Work out the finished part from the listing and answer in its coordinate system (mm). Face numbers are marked on the shaded views. Give positions to 0.01 mm unless a question says otherwise; leave off trailing zeros. Order: outer loops, then holes, each group sorted by start corner. A loop starts at its lowest first (then second) coordinate and runs counter-clockwise, first axis right, second up.
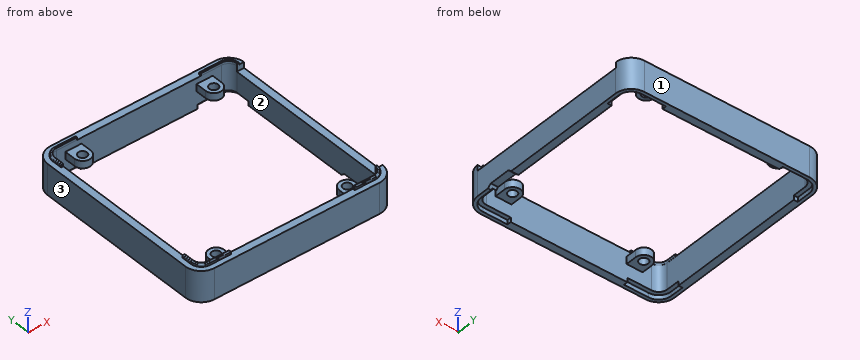
```python
from build123d import *

# Parameters (mm, degrees)
EXTRUDE006_DEPTH                     = 2
EXTRUDE006_ONTO_SKETCH006_ROLL_ANGLE = 90
EXTRUDE006_PLACEMENT_ANGLE           = 90
SKETCH_W                             = 14.047477
SKETCH_H                             = 45.6
EXTRUDE004_DEPTH                     = 10
SKETCH002_R                          = 1.2
EXTRUDE001_DEPTH                     = 2
EXTRUDE005_DEPTH                     = 10
EXTRUDE003_DEPTH                     = 0.7
EXTRUDE003_DEPTH_BACK                = 0.2
FILLET_R                             = 0.2
CHAMFER_SIZE                         = 0.2
EXTRUDE002_DEPTH                     = 2
EXTRUDE_DEPTH                        = 1.6
EXTRUDE_DEPTH_BACK                   = 6.8


with BuildPart() as extrude006:
    # Sketch006 as drawn → Extrude006 (new, symmetric)
    with BuildSketch(Plane.XY):
        Polygon((-3.8, 0), (-2.9, 0.8), (2.9, 0.8), (3.8, 0), align=None)
    extrude(amount=EXTRUDE006_DEPTH, both=True)


with BuildPart() as extrude006_1:
    # Extrude006 onto Sketch006 roll: moved
    add(extrude006.part.rotate(Axis((0, 0, 0), (1, 0, 0)), EXTRUDE006_ONTO_SKETCH006_ROLL_ANGLE))


with BuildPart() as extrude006_2:
    # Extrude006 onto Sketch006 placement: moved
    add(extrude006_1.part)


with BuildPart() as extrude006_3:
    # Extrude006 placement: moved
    add(extrude006_2.part.moved(Location((50, 9.5, -6.8))).rotate(Axis((50, 9.5, -6.8), (0, 0, 1)), EXTRUDE006_PLACEMENT_ANGLE))


with BuildPart() as extrude004:
    # Sketch → Extrude004 (new body)
    with BuildSketch(Plane.XY):
        with Locations((51.252235, 25)):
            Rectangle(SKETCH_W, SKETCH_H)
    extrude(amount=EXTRUDE004_DEPTH)


with BuildPart() as extrude001:
    # Sketch002 → Extrude001 (new body)
    with BuildSketch(Plane.XY):
        with BuildLine():
            Line((4.8, 47), (4.8, 51))
            Line((4.8, 51), (9.2, 51))
            Line((9.2, 51), (9.2, 47.000001))
            ThreePointArc((4.8, 47), (7, 44.8), (9.2, 47.000001))
        make_face()
        with Locations((7, 47)):
            Circle(SKETCH002_R, mode=Mode.SUBTRACT)
        with BuildLine():
            ThreePointArc((9.2, 3), (7, 5.2), (4.8, 3))
            Line((4.8, 3), (4.8, -1))
            Line((4.8, -1), (9.2, -1))
            Line((9.2, -1), (9.2, 3))
        make_face()
        with Locations((7, 3)):
            Circle(SKETCH002_R, mode=Mode.SUBTRACT)
        with BuildLine():
            Line((40.8, 47), (40.8, 51))
            Line((40.8, 51), (45.2, 51))
            Line((45.2, 51), (45.2, 46.999987))
            ThreePointArc((40.8, 47), (42.999993, 44.8), (45.2, 46.999987))
        make_face()
        with Locations((43, 47)):
            Circle(SKETCH002_R, mode=Mode.SUBTRACT)
        with BuildLine():
            ThreePointArc((45.2, 3), (43, 5.2), (40.8, 3))
            Line((40.8, 3), (40.8, -1))
            Line((40.8, -1), (45.2, -1))
            Line((45.2, -1), (45.2, 3))
        make_face()
        with Locations((43, 3)):
            Circle(SKETCH002_R, mode=Mode.SUBTRACT)
    extrude(amount=-EXTRUDE001_DEPTH)


with BuildPart() as extrude005:
    # Sketch005 → Extrude005 (new body)
    with BuildSketch(Plane.XY):
        Polygon((8, 53), (8, 45), (-3, 45), (-3, 5), (8, 5), (8, -3), (42, -3), (42, 5), (53, 5), (53, 45), (42, 45), (42, 53), align=None)
    extrude(amount=EXTRUDE005_DEPTH)


with BuildPart() as cut003:
    # Sketch004 → Extrude003 (new body, two sides)
    with BuildSketch(Plane.XY) as extrude003_sk:
        with BuildLine():
            Line((2.3, 50.6), (47.7, 50.6))
            ThreePointArc((50.6, 47.7), (49.75061, 49.75061), (47.7, 50.6))
            Line((50.6, 47.7), (50.6, 2.3))
            ThreePointArc((47.7, -0.6), (49.75061, 0.24939), (50.6, 2.3))
            Line((47.7, -0.6), (2.3, -0.6))
            ThreePointArc((-0.6, 2.3), (0.24939, 0.24939), (2.3, -0.6))
            Line((-0.6, 2.3), (-0.6, 47.7))
            ThreePointArc((2.3, 50.6), (0.24939, 49.75061), (-0.6, 47.7))
        make_face()
        with BuildLine():
            Line((2.3, 50), (47.7, 50))
            ThreePointArc((50, 47.7), (49.326346, 49.326346), (47.7, 50))
            Line((50, 47.7), (50, 2.3))
            ThreePointArc((47.7, 0), (49.326346, 0.673654), (50, 2.3))
            Line((47.7, 0), (2.3, 0))
            ThreePointArc((0, 2.3), (0.673654, 0.673654), (2.3, 0))
            Line((0, 2.3), (0, 47.7))
            ThreePointArc((2.3, 50), (0.673654, 49.326346), (0, 47.7))
        make_face(mode=Mode.SUBTRACT)
    extrude(amount=EXTRUDE003_DEPTH)
    extrude(extrude003_sk.sketch, amount=-EXTRUDE003_DEPTH_BACK)


with BuildPart() as cut003_1:
    # Extrude003 placement: moved
    add(cut003.part.moved(Location((0, 0, 1.6))))

    # Fillet
    fillet_edges = [cut003_1.edges().sort_by_distance(p)[0] for p in [
        (-0.6, 25, 2.3),
        (0.24939, 49.75061, 2.3),
        (25, 50.6, 2.3),
        (49.75061, 49.75061, 2.3),
        (50.6, 25, 2.3),
        (49.75061, 0.24939, 2.3),
        (25, -0.6, 2.3),
        (0.24939, 0.24939, 2.3),
    ]]
    fillet(fillet_edges, radius=FILLET_R)

    # Chamfer
    chamfer_edges = [cut003_1.edges().sort_by_distance(p)[0] for p in [
        (0, 25, 1.4),
        (0.673654, 49.326346, 1.4),
        (25, 50, 1.4),
        (49.326346, 49.326346, 1.4),
        (50, 25, 1.4),
        (49.326346, 0.673654, 1.4),
        (25, 0, 1.4),
        (0.673654, 0.673654, 1.4),
    ]]
    chamfer(chamfer_edges, length=CHAMFER_SIZE)

    # Cut003: cut Extrude005
    add(extrude005.part, mode=Mode.SUBTRACT)


with BuildPart() as extrude002:
    # Sketch003 → Extrude002 (new body)
    with BuildSketch(Plane.XY):
        with BuildLine():
            Line((2.3, 51.1), (9, 51.1))
            Line((9, 44), (9, 51.1))
            Line((-1.1, 44), (9, 44))
            Line((-1.1, 44), (-1.1, 47.654452))
            ThreePointArc((2.3, 51.1), (-0.12032, 50.088024), (-1.1, 47.654452))
        make_face()
        with BuildLine():
            Line((51.1, 47.699699), (51.1, 44))
            Line((41, 44), (51.1, 44))
            Line((41, 51.1), (41, 44))
            Line((41, 51.1), (47.698586, 51.1))
            ThreePointArc((51.1, 47.699699), (50.103681, 50.104468), (47.698586, 51.1))
        make_face()
        with BuildLine():
            Line((47.6997, -1.1), (41, -1.1))
            Line((41, -1.1), (41, 6))
            Line((41, 6), (51.1, 6))
            Line((51.1, 6), (51.1, 2.297304))
            ThreePointArc((47.6997, -1.1), (50.103016, -0.105134), (51.1, 2.297304))
        make_face()
        with BuildLine():
            Line((-1.1, 2.300296), (-1.1, 6))
            Line((-1.1, 6), (9, 6))
            Line((9, 6), (9, -1.1))
            Line((9, -1.1), (2.294563, -1.1))
            ThreePointArc((-1.1, 2.300296), (-0.106103, -0.10205), (2.294563, -1.1))
        make_face()
    extrude(amount=-EXTRUDE002_DEPTH)


with BuildPart() as extrude002_1:
    # Extrude002 placement: moved
    add(extrude002.part.moved(Location((0, 0, -5.6))))


with BuildPart() as cut004:
    # Sketch001 → Extrude (new body, two sides)
    with BuildSketch(Plane.XY) as extrude_sk:
        with BuildLine():
            Line((2.3, 52), (47.7, 52))
            ThreePointArc((52, 47.7), (50.740559, 50.740559), (47.7, 52))
            Line((52, 47.7), (52, 2.3))
            ThreePointArc((47.7, -2), (50.740559, -0.740559), (52, 2.3))
            Line((47.7, -2), (2.3, -2))
            ThreePointArc((-2, 2.3), (-0.740559, -0.740559), (2.3, -2))
            Line((-2, 2.3), (-2, 47.7))
            ThreePointArc((2.3, 52), (-0.740559, 50.740559), (-2, 47.7))
        make_face()
        with BuildLine():
            Line((2.3, 50.01), (47.7, 50.01))
            ThreePointArc((50.01, 47.7), (49.333417, 49.333417), (47.7, 50.01))
            Line((50.01, 47.7), (50.01, 2.3))
            ThreePointArc((47.7, -0.01), (49.333417, 0.666583), (50.01, 2.3))
            Line((47.7, -0.01), (2.3, -0.01))
            ThreePointArc((-0.01, 2.3), (0.666583, 0.666583), (2.3, -0.01))
            Line((-0.01, 2.3), (-0.01, 47.7))
            ThreePointArc((2.3, 50.01), (0.666583, 49.333417), (-0.01, 47.7))
        make_face(mode=Mode.SUBTRACT)
    extrude(amount=EXTRUDE_DEPTH)
    extrude(extrude_sk.sketch, amount=-EXTRUDE_DEPTH_BACK)

    # Cut002: cut Extrude002
    add(extrude002_1.part, mode=Mode.SUBTRACT)

    # Fusion001: union Cut003
    add(cut003_1.part)

    # Fusion002: union Extrude001
    add(extrude001.part)

    # Cut: cut Extrude004
    add(extrude004.part, mode=Mode.SUBTRACT)

    # Cut004: cut Extrude006
    add(extrude006_3.part, mode=Mode.SUBTRACT)


solid = cut004.part
```
1. The part is cut by section A-A (x = 39.5). Write down the section's boundary in (y, z).
Findings below:
outline: (-2, -6.8) - (-0.01, -6.8) - (-0.01, 1.6) - (-2, 1.6) - close; (50.01, -6.8) - (52, -6.8) - (52, 1.6) - (50.01, 1.6) - close
2. The part is cut by section D-D (x = 7). State how many separate pieces and enclosed holes the cut face has, then the cut area to 3 significant figures.
Findings below:
separate pieces: 4
enclosed holes: 0
area: 42.9 mm2
3. The part is cut by section B-B (y = 42.5). Write down the section's boundary in (x, z), then the cut area to 3 significant figures.
Findings below:
outline: (-2, -6.8) - (-0.01, -6.8) - (-0.01, 1.6) - (-2, 1.6) - close; (50.01, -6.8) - (52, -6.8) - (52, 0) - (50.01, 0) - close
area: 30.2 mm2
4. Given P1, Ø0.9, axis at x = -0.5, z = -6, coming from the -Y side; P2, Ø1.3, axis at x = 42.5, y = 3.5, coming from the +Z side; P3, Ø5.5, axis at x = 5, y = 49, coming from the -Z side; P4, Ø2, axis at y = 49, z = -1, coming from the -X side, each flat-ended and moving along its own axis, determine where each tip first touches the part or whether it passes through.
Findings below:
P1: stops at y = -1.3
P2: stops at z = 0
P3: stops at z = -6.8
P4: stops at x = -1.99
5. Straight lines are drawn through the part: probe 1 along Y at (x, z) = (7, -0.55); probe 2 along X at (y, z) = (37, -4.75). For each, find the intervals that lie inside material, in ascending order.
Findings below:
probe 1: y = -2 to 1.8, 4.2 to 5.2, 44.8 to 45.8, 48.2 to 52
probe 2: x = -2 to -0.01, 50.01 to 52
6. The mould has two halves that part along X. Classify the marked faces 1, 2 and 3: pulls with the +X half, pulls with the -X half, needs draft (parallel to the pull), parting line crosses it, or undercut.
Findings below:
face 1: needs draft
face 2: undercut
face 3: pulls with the -X half
7. The part is cut by section C-C (z = -3.25). Write down the section's boundary in (x, y).
Findings below:
outline: (-2, 2.3) arc R4.3 ccw to (2.3, -2) - (47.7, -2) arc R4.3 ccw to (52, 2.3) - (52, 47.7) arc R4.3 ccw to (47.7, 52) - (2.3, 52) arc R4.3 ccw to (-2, 47.7) - close; hole (-0.01, 2.3) arc R2.31 ccw to (2.3, -0.01) - (47.7, -0.01) arc R2.31 ccw to (50.01, 2.3) - (50.01, 47.7) arc R2.31 ccw to (47.7, 50.01) - (2.3, 50.01) arc R2.31 ccw to (-0.01, 47.7) - close
